from build123d import *

# Parameters (mm, degrees)
SZKIC1_W                    = 264
SZKIC1_H                    = 26
DODANIE_WYCI_GNI_CIE1_DEPTH = 6
SZKIC5_W                    = 40
SZKIC5_H                    = 6
WYTNIJ_WYCI_GNI_CIE3_DEPTH  = 6
SZYK_LINIOWY1_COUNT         = 3
SZYK_LINIOWY1_PITCH         = 91
WYTNIJ_WYCI_GNI_CIE4_DEPTH  = 6
SZYK_LINIOWY2_COUNT         = 2
SZYK_LINIOWY2_PITCH         = 91
PRZENIE_CIAN_1_BY           = 1


with BuildPart() as part:
    # Szkic1 → Dodanie-wyciągnięcie1 (new body)
    with BuildSketch(Plane.XY):
        with Locations((-747.9, 7)):
            Rectangle(SZKIC1_W, SZKIC1_H)
    extrude(amount=-DODANIE_WYCI_GNI_CIE1_DEPTH)

    # Szkic5 → Wytnij-wyciągnięcie3 (cut)
    with BuildSketch(Plane.XY):
        with Locations((-869.9, -3)):
            Rectangle(SZKIC5_W, SZKIC5_H)
    wytnij_wyci_gni_cie3 = extrude(amount=-WYTNIJ_WYCI_GNI_CIE3_DEPTH, mode=Mode.SUBTRACT)

    # Szyk liniowy1: Wytnij-wyciągnięcie3 ×3
    with Locations(*[(i * SZYK_LINIOWY1_PITCH, 0, 0) for i in range(1, SZYK_LINIOWY1_COUNT)]):
        add(wytnij_wyci_gni_cie3, mode=Mode.SUBTRACT)

    # Szkic6 → Wytnij-wyciągnięcie4 (cut)
    with BuildSketch(Plane.XY):
        Polygon((-777.35, 0), (-780.45, 0), (-780.45, 4), (-781.825, 4), (-781.825, 6), (-780.45, 6), (-780.45, 6.5), (-777.35, 6.5), (-777.35, 6), (-775.975, 6), (-775.975, 4), (-777.35, 4), align=None)
    wytnij_wyci_gni_cie4 = extrude(amount=-WYTNIJ_WYCI_GNI_CIE4_DEPTH, mode=Mode.SUBTRACT)

    # Szyk liniowy2: Wytnij-wyciągnięcie4 ×2
    with Locations(*[(i * SZYK_LINIOWY2_PITCH, 0, 0) for i in range(1, SZYK_LINIOWY2_COUNT)]):
        add(wytnij_wyci_gni_cie4, mode=Mode.SUBTRACT)

    # Przenieś ścianę1: a face moved inward by 1.0
    extrude(part.faces().sort_by_distance((-879.9, 10, -3))[0], amount=PRZENIE_CIAN_1_BY, dir=(1, 0, 0), mode=Mode.SUBTRACT)


solid = part.part
Design review of the part built by this model. Coordinates are the model's own, in mm. A direction names the side the tool comes from. Coordinates: 2 decimals unless noted, no trailing zeros. Loops run counter-clockwise (first coordinate to the right, second up) from the corner with the lowest first, then second, coordinate; pieces in that order, holes last. Notation, with made-up numbers: (65, -7.5) -> (105, -7.5) arc R15 ccw to (105, 2.5) -> close; hole circle Ø3 at (-15, -36). An arc over 180 degrees is marked (long way). Use a Markdown table: item, result. Add a question column.
Item 1: We need section A-A, the plane y = -3.75. Write out the cut boundary in (x, z), and give its area (3 significant figures).
Item 2: Machinability: for faces 1 (the flat face through (-642, -6, -3)), 2 (the flat face through (-865, 0, -3)), 3 (the flat face through (-707.9, -3, -3)), which of the approach directions +Z, -Z, +X, -X, +Y, -Y give a long, thin tool a straight path to every point of the face, cutting with its end or side? Answer none if there is none.
Item 3: We need section B-B, the plane x = -698. Write out the cut boundary in (y, z), and give its area (3 significant figures).
Item 4: Wall thickness on L1, parallel to X at y = 3, z = -0.2; L2, parallel to X at y = -3.75, z = -0.9; L3, parallel to Y at x = -697.5, z = -4.3: over which ranges is each line inside the solid? List them lowest first. Write a range as from..to.
Item 5: Clearance check with flat-ended pins moving along their axes: P1, Ø3, axis at x = -701.5, z = -3, coming from the -Y side; P2, Ø1.8, axis at y = -4.5, z = -2, coming from the -X side. State where each tip first meets the part, or that it passes through.
Item 6: The part is to be moulded in two halves that separate along X. For faces 4 (the flat face through (-677, 0, -3)), 5 (the flat face through (-749, 7, -6)), 6 (the flat face through (-615.9, 7, -3)), 7 (the flat face through (-849.9, -3, -3)), say which applies: +X half, -X half, draft (parallel to the pull), parting line (faces both ways), or undercut.
Numbers:
| question | item | result |
|---|---|---|
| 1 | outline | (-849.9, -6) -> (-798.9, -6) -> (-798.9, 0) -> (-849.9, 0) -> close; (-758.9, -6) -> (-707.9, -6) -> (-707.9, 0) -> (-758.9, 0) -> close; (-667.9, -6) -> (-615.9, -6) -> (-615.9, 0) -> (-667.9, 0) -> close |
| 1 | area | 924 mm^2 |
| 2 | face 1 | +Z, -Z, +X, -X, -Y |
| 2 | face 2 | +Z, -Z, -X, -Y |
| 2 | face 3 | +Z, -Z, -Y |
| 3 | outline | (0, -6) -> (20, -6) -> (20, 0) -> (0, 0) -> close |
| 3 | area | 120 mm^2 |
| 4 | L1 | x = -878.9..-780.45, -777.35..-689.45, -686.35..-615.9 |
| 4 | L2 | x = -849.9..-798.9, -758.9..-707.9, -667.9..-615.9 |
| 4 | L3 | y = 0..20 |
| 5 | P1 | stops at y = 0 |
| 5 | P2 | stops at x = -849.9 |
| 6 | face 4 | undercut |
| 6 | face 5 | draft |
| 6 | face 6 | +X half |
| 6 | face 7 | -X half |
